```python
from build123d import *

# Parameters (mm, degrees)
SKETCH001_W  = 74
SKETCH001_H  = 43
SKETCH001_R  = 1.05
PAD_DEPTH    = 2.5
SKETCH_R     = 2.5
SKETCH_R_2   = 1.05
PAD001_DEPTH = 7
FILLET_R     = 2


with BuildPart() as part:
    # Sketch001 → Pad (new body)
    with BuildSketch(Plane.XY):
        Rectangle(SKETCH001_W, SKETCH001_H)
        with Locations((-29, -13.5)):
            Circle(SKETCH001_R, mode=Mode.SUBTRACT)
        with Locations((29, -13.5)):
            Circle(SKETCH001_R, mode=Mode.SUBTRACT)
        with Locations((29, 13.5)):
            Circle(SKETCH001_R, mode=Mode.SUBTRACT)
        with Locations((-29, 13.5)):
            Circle(SKETCH001_R, mode=Mode.SUBTRACT)
    extrude(amount=PAD_DEPTH)

    # Sketch → Pad001 (join)
    with BuildSketch(Plane.XY):
        with Locations((-29, 13.5)):
            Circle(SKETCH_R)
        with Locations((-29, 13.5)):
            Circle(SKETCH_R_2, mode=Mode.SUBTRACT)
        with Locations((-29, -13.5)):
            Circle(SKETCH_R)
        with Locations((-29, -13.5)):
            Circle(SKETCH_R_2, mode=Mode.SUBTRACT)
        with Locations((29, -13.5)):
            Circle(SKETCH_R)
        with Locations((29, -13.5)):
            Circle(SKETCH_R_2, mode=Mode.SUBTRACT)
        with Locations((29, 13.5)):
            Circle(SKETCH_R)
        with Locations((29, 13.5)):
            Circle(SKETCH_R_2, mode=Mode.SUBTRACT)
    extrude(amount=PAD001_DEPTH)

    # Fillet
    fillet_edges = [part.edges().sort_by_distance(p)[0] for p in [
        (-37, 0, 2.5),
        (0, 21.5, 2.5),
        (0, -21.5, 2.5),
        (37, 0, 2.5),
        (-31.5, -13.5, 2.5),
        (26.5, -13.5, 2.5),
        (-31.5, 13.5, 2.5),
        (26.5, 13.5, 2.5),
    ]]
    fillet(fillet_edges, radius=FILLET_R)


solid = part.part
```
Read the model definition and answer for the solid it produces. Units are mm, in the model's axes. A direction names the side the tool comes from. Give positions to 0.01 mm unless a question says otherwise; leave off trailing zeros. Write each loop counter-clockwise with the first axis right and the second up, starting at its lowest first coordinate (ties: lowest second). Pieces come first, ordered by that corner, then holes. Notation, with made-up numbers: (48.25, 26) -> (78.25, 26) arc R15 ccw to (78.25, 39) -> close; hole circle Ø10 at (57, 44.25). An arc over 180 degrees is marked (long way). Answer in a Markdown table with one row per item.
1) Section D-D on y = -4.5 is taken. Give the vertices of the cut face in (x, z).
Results list:
| item | result |
|---|---|
| outline | (-37, 0) -> (37, 0) -> (37, 0.5) arc R2 ccw to (35, 2.5) -> (-35, 2.5) arc R2 ccw to (-37, 0.5) -> close |
2) Determine the mould class of faces 3 (the cylindrical face through (0.52, -20.9, 1.93)), 4 (the cylindrical face through (29.56, -12.61, 3.45)), 5 (the cylindrical face through (36.4, 0.3, 1.93)) for opening direction X: released by +X, released by -X, zero draft, split by the parting line, or undercut.
Results list:
| item | result |
|---|---|
| face 3 | zero draft |
| face 4 | undercut |
| face 5 | released by +X |
3) Straight lines are drawn through the part: line 1 (Y direction, x = -29, z = 5.5); line 2 (Z direction, x = 19, y = 9.5); line 3 (Y direction, x = 29, z = 3.5). For each, find the intervals that lie inside material, in ascending order. Write a range as [from, to].
Results list:
| item | result |
|---|---|
| line 1 | [-16, -14.55], [-12.45, -11], [11, 12.45], [14.55, 16] |
| line 2 | [0, 2.5] |
| line 3 | [-16.27, -14.55], [-12.45, -10.73], [10.73, 12.45], [14.55, 16.27] |
4) A tool of negligible diameter and unlimited length cuts with its end or side. For faces 1 (the flat face through (-29, 12, 7)), 2 (the cylindrical face through (-29.54, 11.06, 5.73)), from which of +Z, -Z, +X, -X, +Y, -Y can it reach the whole face along a straight path? Write none if from no direction.
Results list:
| item | result |
|---|---|
| face 1 | +Z, +X, -X, +Y, -Y |
| face 2 | +Z |
5) Section C-C on x = 29 is taken. Give the vertices of the cut face in (y, z).
Results list:
| item | result |
|---|---|
| outline | (-21.5, 0) -> (-14.55, 0) -> (-14.55, 7) -> (-16, 7) -> (-16, 4.5) arc R2 cw to (-18, 2.5) -> (-19.5, 2.5) arc R2 ccw to (-21.5, 0.5) -> close; (-12.45, 0) -> (12.45, 0) -> (12.45, 7) -> (11, 7) -> (11, 4.5) arc R2 cw to (9, 2.5) -> (-9, 2.5) arc R2 cw to (-11, 4.5) -> (-11, 7) -> (-12.45, 7) -> close; (14.55, 0) -> (21.5, 0) -> (21.5, 0.5) arc R2 ccw to (19.5, 2.5) -> (18, 2.5) arc R2 cw to (16, 4.5) -> (16, 7) -> (14.55, 7) -> close |
6) Section A-A on z = 5.5 is taken. Give the vertices of the cut face in (x, y).
Results list:
| item | result |
|---|---|
| outline | circle Ø5 at (-29, -13.5); circle Ø5 at (-29, 13.5); circle Ø5 at (29, -13.5); circle Ø5 at (29, 13.5); hole circle Ø2.1 at (-29, -13.5); hole circle Ø2.1 at (-29, 13.5); hole circle Ø2.1 at (29, -13.5); hole circle Ø2.1 at (29, 13.5) |
7) Section B-B on y = 13.5 is taken. Give the vertices of the cut face in (x, z), plus the area to 3 significant figures.
Results list:
| item | result |
|---|---|
| outline | (-37, 0) -> (-30.05, 0) -> (-30.05, 7) -> (-31.5, 7) -> (-31.5, 4.5) arc R2 cw to (-33.5, 2.5) -> (-35, 2.5) arc R2 ccw to (-37, 0.5) -> close; (-27.95, 0) -> (27.95, 0) -> (27.95, 7) -> (26.5, 7) -> (26.5, 4.5) arc R2 cw to (24.5, 2.5) -> (-24.5, 2.5) arc R2 cw to (-26.5, 4.5) -> (-26.5, 7) -> (-27.95, 7) -> close; (30.05, 0) -> (37, 0) -> (37, 0.5) arc R2 ccw to (35, 2.5) -> (33.5, 2.5) arc R2 cw to (31.5, 4.5) -> (31.5, 7) -> (30.05, 7) -> close |
| area | 202 mm^2 |
8) Each of these flat-tipped pins is pushed along its axis until it touches: pin 1 Ø11.5 at (x, y) = (15.5, -2) entering from +Z; pin 2 Ø1.5 at (y, z) = (8.5, 1.5) entering from +X; pin 3 Ø1 at (y, z) = (0.5, 1.5) entering from -X; pin 4 Ø3.5 at (x, y) = (-29, 13.5) entering from -Z. Where does it stop, or does it pass through?
Results list:
| item | result |
|---|---|
| pin 1 | z = 2.5 |
| pin 2 | x = 36.98 |
| pin 3 | x = -36.94 |
| pin 4 | z = 0 |
